For this review, use the dimensioned drawing (mm, ordinates from the lowest corner) and the shaded views. A direction names the side the tool comes from. Coordinates: 2 decimals unless noted, no trailing zeros. Write each loop counter-clockwise with the first axis right and the second up, starting at its lowest first coordinate (ties: lowest second). Pieces come first, ordered by that corner, then holes. Notation, with made-up numbers: M 84,78.5 L 122,78.5 A35 cw 122,113.5 Z; hole C 4.5,20 d2. An arc over 180 degrees is marked long. One line per question, with ' | ' between items.
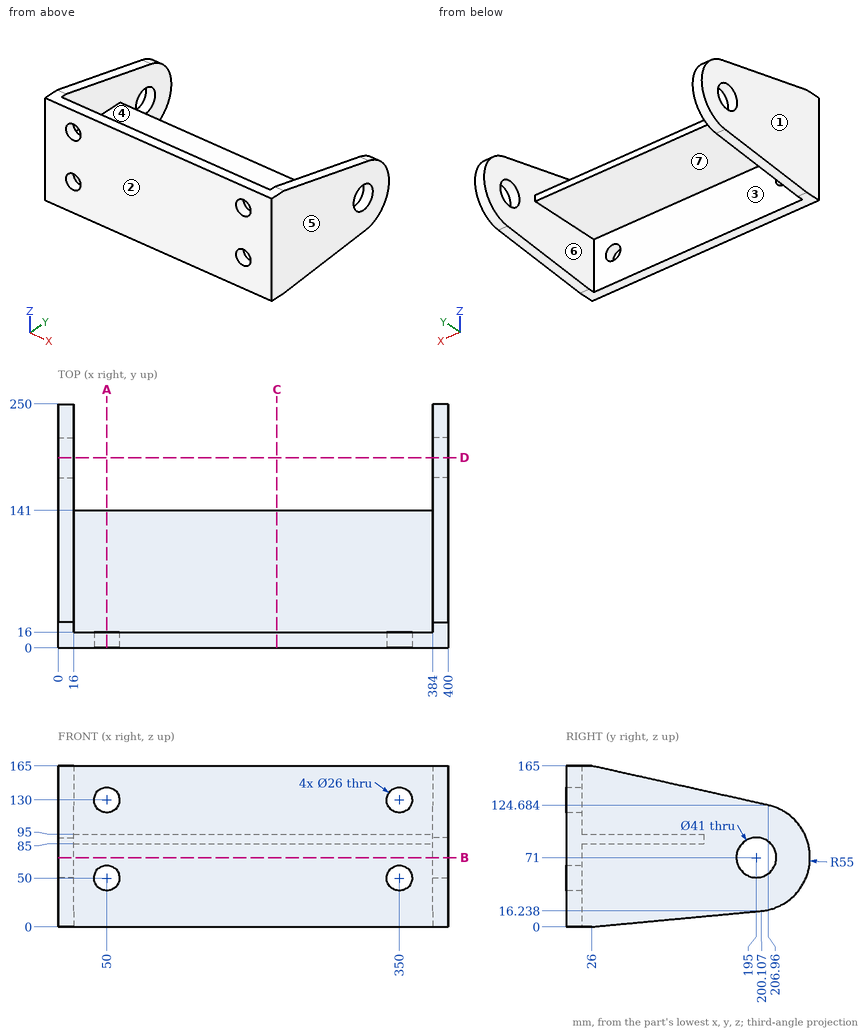
1. Take a section at B-B (z = 71). Write out the cut boundary in (x, y), then the cut area to 3 significant figures.
Answer sheet:
outline: M 0,0 L 400,0 L 400,174.5 L 384,174.5 L 384,16 L 16,16 L 16,174.5 L 0,174.5 Z; M 0,215.5 L 16,215.5 L 16,250 L 0,250 Z; M 384,215.5 L 400,215.5 L 400,250 L 384,250 Z | area: 12,600 mm^2
2. Insertion check: pin 1 Ø5 at (x, z) = (182, 90.5) entering from +Y; pin 2 Ø2 at (x, z) = (283, 29) entering from +Y. Each pin has a flat end and moves straight along its axis. Give the tip position at first contact, or say it passes through.
Answer sheet:
pin 1: y = 141 | pin 2: y = 16
3. Take a section at D-D (y = 195). Write out the cut boundary in (x, z).
Answer sheet:
outline: M 0,15.76 L 16,15.76 L 16,50.5 L 0,50.5 Z; M 0,91.5 L 16,91.5 L 16,127.35 L 0,127.35 Z; M 384,15.76 L 400,15.76 L 400,50.5 L 384,50.5 Z; M 384,91.5 L 400,91.5 L 400,127.35 L 384,127.35 Z
4. Take a section at C-C (x = 224.5). Write out the cut boundary in (y, z), then the cut area to 3 significant figures.
Answer sheet:
outline: M 0,0 L 16,0 L 16,85 L 141,85 L 141,95 L 16,95 L 16,165 L 0,165 Z | area: 3,890 mm^2
5. Tool access review of the marked faces 4, 5, 6 and 7: name each direction out of +Z, -Z, +X, -X, +Y, -Y from which nothing blocks a thin tool from reaching the whole face with its end or side.
Answer sheet:
face 4: +Z, +Y | face 5: +Z, -Z, +X, +Y, -Y | face 6: +Y | face 7: -Z, +Y
6. Draft analysis for pull direction X (two halves, no side actions). For the marked faces 1, 2 and 3, state which applies: pulls with the +X half, pulls with the -X half, needs draft (parallel to the pull), parting line crosses it, or undercut.
Answer sheet:
face 1: pulls with the -X half | face 2: needs draft | face 3: undercut
7. Take a section at A-A (x = 50). Write out the cut boundary in (y, z).
Answer sheet:
outline: M 0,0 L 16,0 L 16,37 L 0,37 Z; M 0,63 L 16,63 L 16,85 L 141,85 L 141,95 L 16,95 L 16,117 L 0,117 Z; M 0,143 L 16,143 L 16,165 L 0,165 Z
8. To check wall thickness, follow line 1 along X through (y, z) = (11, 130); line 2 along X through (y, z) = (105.5, 69.5); line 3 along Y through (x, z) = (348, 33.5). State the ranges of each line that lie inside material, in increasing order. Write a range as [from, to].
Answer sheet:
line 1: [0, 37], [63, 337], [363, 400] | line 2: [0, 16], [384, 400] | line 3: [0, 16]
